The listing builds one solid part. Answer for the finished solid, in the listing's coordinates (mm). A direction names the side the tool comes from. Coordinates: 2 decimals unless noted, no trailing zeros. Write each loop counter-clockwise with the first axis right and the second up, starting at its lowest first coordinate (ties: lowest second). Pieces come first, ordered by that corner, then holes. Notation, with made-up numbers: M 4.25,-1.75 L 47.25,-1.75 A13 cw 47.25,5.25 Z; hole C -24,21.5 d7. An arc over 180 degrees is marked long. Answer as CSV lines item,"result".
```python
from build123d import *

# Parameters (mm, degrees)
F0_W     = 77.7875
F0_H     = 31.75
F1_DEPTH = 3.175
F3_R     = 2.2098
F4_DEPTH = 25.4


with BuildPart() as f1:
    # F0 (on Front) → F1 (new body)
    with BuildSketch(Plane.XZ):
        with Locations((-0.282224, 31.94195)):
            Rectangle(F0_W, F0_H)
        with Locations((77.505276, 31.94195)):
            Rectangle(F0_W, F0_H)
    extrude(amount=F1_DEPTH)

    # F3 (on face) → F4 (join)
    with BuildSketch(Plane.XZ.offset(3.175)):
        with Locations((38.613036, 31.945616)):
            Circle(F3_R)
    extrude(amount=F4_DEPTH)


solid = f1.part
```
Q1. Find section A-A (x = 39). Give the vertices of the cut face in (y, z) (3 decimals).
Output:
outline,"M -28.575,29.77 L -3.175,29.77 L -3.175,16.067 L 0,16.067 L 0,47.817 L -3.175,47.817 L -3.175,34.121 L -28.575,34.121 Z"
Q2. Find section C-C (y = -23.75). Give the vertices of the cut face in (x, z), and give its area (3 significant figures).
Output:
outline,"C 38.61,31.95 d4.42"
area,"15.3 mm2"
Q3. For faces 1 (the flat face through (38, -2, 16.067)), 2 (the cylindrical face through (40.72, -15.7, 32.61)), determine the directions among +Z, -Z, +X, -X, +Y, -Y from which every point of the face is accessible in a straight line to the end or side of a thin tool.
Output:
face 1,"-Z, +X, -X, +Y, -Y"
face 2,"-Y"
Q4. Straight lines are drawn through the part: line 1 (Y direction, x = 47.5, z = 21) (3 decimals); line 2 (X direction, y = -20, z = 30); line 3 (X direction, y = -10.5, z = 33). For each, find the intervals that lie inside material, in ascending order.
Output:
line 1,"-3.175 to 0"
line 2,"37.57 to 39.66"
line 3,"36.67 to 40.56"
Q5. Flat-ended cylindrical pins translate along their axes: pin 1 Ø12 at (y, z) = (-20, 22.5) entering from -X; pin 2 Ø5 at (x, z) = (37.5, 40) entering from -Y (3 decimals). Find the tip coordinate at first contact, or state that the pin passes through.
Output:
pin 1,"through"
pin 2,"y = -3.175"
Q6. Find section D-D (x = -7.5). Give the vertices of the cut face in (y, z) (3 decimals), and give its area (3 significant figures).
Output:
outline,"M -3.175,16.067 L 0,16.067 L 0,47.817 L -3.175,47.817 Z"
area,"101 mm2"
Q7. Find section B-B (z = 44.5). Give the vertices of the cut face in (x, y) (3 decimals).
Output:
outline,"M -39.176,-3.175 L 116.399,-3.175 L 116.399,0 L -39.176,0 Z"
